Build history of the part. All positions in model axes, mm. A direction names the side the tool comes from. Give positions to 0.01 mm unless a question says otherwise; leave off trailing zeros. Loops run counter-clockwise (first coordinate to the right, second up) from the corner with the lowest first, then second, coordinate; pieces in that order, holes last. Notation, with made-up numbers: M -25.75,4 L 32.25,4 A11 ccw 32.25,16 Z; hole C 16,67.25 d10. An arc over 180 degrees is marked long. Put each result on its own line as item: value.
```python
from build123d import *

# Parameters (mm, degrees)
SKETCH1_R           = 1.5
SKETCH1_R_2         = 4.25
SKETCH1_R_3         = 1
BOSS_EXTRUDE2_DEPTH = 5


with BuildPart() as part:
    # Sketch1 → Boss-Extrude2 (new body)
    with BuildSketch(Plane.XY):
        with BuildLine():
            Line((45.25091594, -25.207708346), (50.00091594, -20.457708346))
            Line((50.00091594, -20.457708346), (50.00091594, 24.688738263))
            Line((50.00091594, 24.688738263), (45.147362549, 29.542291654))
            Line((45.147362549, 29.542291654), (26.35446933, 29.542291654))
            Line((26.35446933, 29.542291654), (21.25091594, 24.438738263))
            Line((21.25091594, 24.438738263), (21.25091594, 18.042291654))
            Line((21.25091594, 18.042291654), (20.408095363, 18.042291654))
            Line((20.408095363, 18.042291654), (16.70086026, 18.042291654))
            ThreePointArc((16.70086026, 18.042291654), (12.892426636, 17.542145454), (9.3422674, 16.075624987))
            ThreePointArc((9.3422674, 16.075624987), (2.182128173, 13.100539865), (-5.49908406, 12.043324729))
            Line((-5.49908406, 12.043324729), (-5.49908406, 12.039085999))
            ThreePointArc((-5.49908406, 12.039085999), (-15.49908406, 2.292291654), (-5.49908406, -7.454502691))
            Line((-5.49908406, -7.454502691), (-5.49908406, -7.458741422))
            ThreePointArc((-5.49908406, -7.458741422), (2.182128173, -8.515956557), (9.3422674, -11.491041679))
            ThreePointArc((9.3422674, -11.491041679), (12.892426636, -12.957562146), (16.70086026, -13.457708346))
            Line((16.70086026, -13.457708346), (20.408095363, -13.457708346))
            Line((20.408095363, -13.457708346), (21.25091594, -13.457708346))
            Line((21.25091594, -13.457708346), (21.25091594, -20.207708346))
            Line((21.25091594, -20.207708346), (26.25091594, -25.207708346))
            Line((26.25091594, -25.207708346), (45.25091594, -25.207708346))
        make_face()
        with Locations((46.75091594, -7.707708346)):
            Circle(SKETCH1_R, mode=Mode.SUBTRACT)
        with Locations((46.75091594, 12.292291654)):
            Circle(SKETCH1_R, mode=Mode.SUBTRACT)
        with Locations((33.50091594, 14.792291654)):
            Circle(SKETCH1_R_2, mode=Mode.SUBTRACT)
        with Locations((33.50091594, -10.207708346)):
            Circle(SKETCH1_R_2, mode=Mode.SUBTRACT)
        with Locations((19.25091594, 12.292291654)):
            Circle(SKETCH1_R, mode=Mode.SUBTRACT)
        with Locations((19.25091594, -7.707708346)):
            Circle(SKETCH1_R, mode=Mode.SUBTRACT)
        with Locations((-5.74908406, 2.292291654)):
            Circle(SKETCH1_R, mode=Mode.SUBTRACT)
        with Locations((1.25091594, 2.354746229)):
            Circle(SKETCH1_R_3, mode=Mode.SUBTRACT)
        with Locations((-0.755373293, -2.613098521)):
            Circle(SKETCH1_R_3, mode=Mode.SUBTRACT)
        with Locations((-5.686629485, -4.707708346)):
            Circle(SKETCH1_R_3, mode=Mode.SUBTRACT)
        with Locations((-10.654474236, -2.701419114)):
            Circle(SKETCH1_R_3, mode=Mode.SUBTRACT)
        with Locations((-12.74908406, 2.229837079)):
            Circle(SKETCH1_R_3, mode=Mode.SUBTRACT)
        with Locations((-10.742794828, 7.197681829)):
            Circle(SKETCH1_R_3, mode=Mode.SUBTRACT)
        with Locations((-5.811538636, 9.292291654)):
            Circle(SKETCH1_R_3, mode=Mode.SUBTRACT)
        with Locations((-0.843693885, 7.286002421)):
            Circle(SKETCH1_R_3, mode=Mode.SUBTRACT)
    extrude(amount=BOSS_EXTRUDE2_DEPTH)


solid = part.part
```
Q1. Slice it at A-A (y = 13). List the corners of the cut face in (x, z).
Here are the results:
outline: M 1.8,0 L 17.93,0 L 17.93,5 L 1.8,5 Z; M 20.57,0 L 29.65,0 L 29.65,5 L 20.57,5 Z; M 37.35,0 L 45.43,0 L 45.43,5 L 37.35,5 Z; M 48.07,0 L 50,0 L 50,5 L 48.07,5 Z
Q2. Slice it at B-B (x = 46.5). List the corners of the cut face in (y, z).
Here are the results:
outline: M -23.96,0 L -9.19,0 L -9.19,5 L -23.96,5 Z; M -6.23,0 L 10.81,0 L 10.81,5 L -6.23,5 Z; M 13.77,0 L 28.19,0 L 28.19,5 L 13.77,5 Z
Q3. Tool access for faces 1 (the flat face through (36, -25.208, 2)), 2 (the flat face through (19, -13.458, 2)), 3 (the flat face through (19, 18.042, 2)): list every direction of +Z, -Z, +X, -X, +Y, -Y with a clear straight run to the whole face (end or side of a thin tool).
Here are the results:
face 1: +Z, -Z, +X, -X, -Y
face 2: +Z, -Z, -X, -Y
face 3: +Z, -Z, -X, +Y
Q4. Slice it at D-D (y = 26.5). List the corners of the cut face in (x, z).
Here are the results:
outline: M 23.31,0 L 48.19,0 L 48.19,5 L 23.31,5 Z
Q5. Slice it at C-C (z = 0.7). State how many separate pieces and enclosed holes the cut face has, and give its area (3 significant figures).
Here are the results:
separate pieces: 1
enclosed holes: 15
area: 2,200 mm²
Q6. Drop flat-ended pins along their axis: pin 1 Ø1.2 at (x, y) = (-0.84, 7.29) entering from +Z; pin 2 Ø2.5 at (x, z) = (18.5, 1.5) entering from +Y; pin 3 Ø1 at (x, z) = (21, 1) entering from +Y; pin 4 Ø1.5 at (x, z) = (23.5, 1.5) entering from -Y. Give the stop position or say it passes through.
Here are the results:
pin 1: through
pin 2: y = 18.04
pin 3: y = 24.69
pin 4: y = -23.21
Q7. Mould opens along X. For faces 4 (the flat face through (47.61, 27.08, 2.46)), 5 (the flat face through (21.251, 21, 2)), 6 (the cylindrical face through (-11.795, 2.53, 2.465)), 7 (the cylindrical face through (48.182, 12.743, 2.465)) say: pulls with the +X half, pulls with the -X half, needs draft (parallel to the pull), parting line crosses it, or undercut.
Here are the results:
face 4: pulls with the +X half
face 5: pulls with the -X half
face 6: undercut
face 7: undercut
Q8. Probe line 1 (Y direction, x = 34, z = 0.6); line 2 (Y direction, x = 18, z = 4.7); line 3 (X direction, y = 8, z = 2.15). List the from-to ranges inside material, lowest first. Write a range as from..to.
Here are the results:
line 1: -25.21..-14.43, -5.99..10.57, 19.01..29.54
line 2: -13.46..-8.54, -6.88..11.46, 13.12..18.04
line 3: -13.65..-11.34, -10.15..-1.54, -0.14..50
